Autodesk Inventor part; units mm, degrees
ref_plane "Work Plane1" through (-21.8189, 29, 8.1) normal (0, 1, 0) x (0, 0, 1)
ref_plane "Work Plane2" through (-21.8189, 19, 8.1) normal (0, 0, -1) x (0, 1, 0)
ref_plane "YZ Plane" through (0, 0, 0) normal (1, 0, 0) x (0, 1, 0)
sketch "Sketch1" plane through (0, 0, 0) normal (0, 0, 1) x (1, 0, 0)
  line L0 (5.8439, -14.5) -> (6.8, -14.5)
  line L1 (6.8, -5.5) -> (6.8, -14.5)
  line L2 (6.8, -5.5) -> (5.8439, -5.5)
  arc A0 (5.8439, -3.1) -> (5.8439, -5.5) centre (4, -4.3) ccw
  line L3 (5.8439, -3.1) -> (6.8, -3.1)
  line L4 (6.8, 0) -> (6.8, -3.1)
  line L5 (0, 0) -> (6.8, 0)
  line L6 (0, -20) -> (0, 0)
  line L7 (0, -20) -> (6.8, -20)
  line L8 (6.8, -16.9) -> (6.8, -20)
  line L9 (6.8, -16.9) -> (5.8439, -16.9)
  arc A1 (5.8439, -14.5) -> (5.8439, -16.9) centre (4, -15.7) ccw
  line L10 (-47.1, -14.5) -> (-46.1439, -14.5)
  arc A2 (-46.1439, -16.9) -> (-46.1439, -14.5) centre (-44.3, -15.7) ccw
  line L11 (-46.1439, -16.9) -> (-47.1, -16.9)
  line L12 (-47.1, -16.9) -> (-47.1, -20)
  line L13 (-40.3, -20) -> (-47.1, -20)
  line L14 (-40.3, 0) -> (-40.3, -20)
  line L15 (-40.3, 0) -> (-47.1, 0)
  line L16 (-47.1, 0) -> (-47.1, -3.1)
  line L17 (-47.1, -3.1) -> (-46.1439, -3.1)
  arc A3 (-46.1439, -5.5) -> (-46.1439, -3.1) centre (-44.3, -4.3) ccw
  line L18 (-46.1439, -5.5) -> (-47.1, -5.5)
  line L19 (-47.1, -5.5) -> (-47.1, -14.5)
extrude "Extrusion1" add sketch "Sketch1" along normal blind 4
sketch "Sketch2" plane through (0, 0, 0) normal (0, 1, 0) x (1, 0, 0)
  line L0 (0, 0) -> (6.8, 0)
  line L1 (0, 0) -> (0, -4)
  line L2 (6.8, -4) -> (0, -4)
  line L3 (6.8, 0) -> (6.8, -4)
  line L4 (-47.1, 0) -> (-47.1, -4)
  line L5 (-40.3, -4) -> (-47.1, -4)
  line L6 (6.8, 0) -> (-47.1, 0)
  line L7 (-47.1, 0) -> (-47.1, -4)
  line L8 (-47.1, -4) -> (6.8, -4)
  line L9 (6.8, -4) -> (6.8, 0)
extrude "Extrusion2" add sketch "Sketch2" along normal blind 4 contours L1 L8 L5 L4 L6
sketch "Sketch3" plane through (0, 0, 4) normal (1, 0, 0) x (0, 0, -1)
  line L0 (4, 0) -> (0, 0)
  line L1 (4, 4) -> (4, 0)
  line L2 (0, 4) -> (4, 4)
  line L3 (0, 0) -> (0, 4)
extrude "Extrusion3" add sketch "Sketch3" along normal up to surface (6.8 mm away)
sketch "Sketch4" plane through (0, 4, 0) normal (0, 1, 0) x (1, 0, 0)
  line L0 (6.8, 0) -> (-47.1, 0)
  line L1 (-47.1, -4) -> (6.8, -4)
  line L2 (-9.3767, -8.1) -> (-9.3767, -13.1) construction
  line L3 (-21.8189, -8.1) -> (-9.3767, -8.1) construction
  arc A0 (-17.3767, -8.1) -> (-40.8, 16.4941) centre (-48.3, -14.1) ccw construction
  line L4 (-9.3767, -4) -> (-16.3767, -4) construction
  line L5 (-16.3767, -4) -> (-16.3767, -8.1) construction
  line L6 (-16.3767, -8.1) -> (-9.3767, -8.1) construction
  line L7 (-9.3767, -8.1) -> (-9.3767, -4) construction
  line L8 (-9.3767, -4) -> (-16.3767, -4)
  line L9 (-16.3767, -4) -> (-16.3767, 0)
  line L10 (-16.3767, 0) -> (-9.3767, 0)
  line L11 (-9.3767, 0) -> (-9.3767, -4)
  point P0 (0, 0)
  dimension "d6" = 7
ref_plane "Work Plane1" through (-21.8189, 29, 8.1) normal (0, 1, 0) x (0, 0, 1)
extrude "Extrusion4" add sketch "Sketch4" along normal up to surface (25 mm away)
sketch "Sketch5" plane through (0, 0, 4) normal (0, 0, 1) x (1, 0, 0)
  circle A0 centre (-13.3767, 24) radius 2 construction
  line L0 (-21.8189, 24) -> (-17.3767, 24) construction
  line L1 (-21.8189, 24) -> (-21.8189, 29) construction
  line L2 (-21.8189, 29) -> (-9.3767, 29) construction
  line L3 (-9.3767, 19) -> (-9.3767, 29) construction
  line L4 (-17.3767, 19) -> (-9.3767, 19) construction
  line L5 (-17.3767, 24) -> (-17.3767, 19) construction
  line L6 (-9.3767, 19) -> (-16.3767, 19) construction
  line L7 (-16.3767, 19) -> (-16.3767, 29) construction
  line L8 (-16.3767, 29) -> (-9.3767, 29) construction
  line L9 (-9.3767, 29) -> (-9.3767, 19) construction
  line L10 (-9.3767, 19) -> (-16.3767, 19)
  line L11 (-16.3767, 19) -> (-16.3767, 29)
  line L12 (-16.3767, 29) -> (-9.3767, 29)
  line L13 (-9.3767, 29) -> (-9.3767, 19)
  circle A1 centre (-13.3767, 24) radius 2
ref_plane "Work Plane2" through (-21.8189, 19, 8.1) normal (0, 0, -1) x (0, 1, 0)
extrude "Extrusion5" add sketch "Sketch5" along normal up to surface (4.1 mm away)
fillet "Fillet2" radius 2 2 edges at (-9.3767, 4, 2) (-16.3767, 4, 2)
sketch "Sketch6" plane through (-16.3767, 19, 8.1) normal (-1, 0, 0) x (0, 0, 1)
  line L0 (0, 5) -> (-24.5941, 5) construction
  line L1 (0, 0) -> (-24.5941, 0) construction
  line L2 (-8.1, 10) -> (0.5132, 10) construction
  line L3 (0.5132, 10) -> (0.5132, 5) construction
  line L4 (0.5132, 5) -> (-8.1, 5) construction
  line L5 (-8.1, 5) -> (-8.1, 10) construction
  line L6 (-8.1, 10) -> (0, 10)
  line L7 (0, 10) -> (0, 5)
  line L8 (0, 5) -> (-8.1, 5)
  line L9 (-8.1, 5) -> (-8.1, 10)
  point P0 (-8.1, -19)
extrude "Extrusion6" add sketch "Sketch6" along normal blind 5
sketch "Sketch7" plane through (-16.3767, 24, 0) normal (0, -1, 0) x (1, 0, 0)
  line L0 (0, 8.1) -> (0, 0)
  line L1 (0, 8.1) -> (-5, 8.1)
  line L2 (-5, 0) -> (-5, 8.1)
  line L3 (0, 0) -> (-5, 0)
  point P0 (16.3767, 0)
extrude "Extrusion7" cut sketch "Sketch7" against normal blind 0.4
sketch "Sketch8" plane through (0, 0, 0) normal (0, 0, -1) x (-1, 0, 0)
  circle A0 centre (13.3767, 24) radius 2 construction
  circle A1 centre (13.3767, 24) radius 2
extrude "Extrusion8" cut sketch "Sketch8" against normal blind 4
fillet "Fillet3" radius 1 1 edges at (-16.3767, 24.4, 4.05)
sketch "Sketch9" plane through (-9.3767, 19, 8.1) normal (1, 0, 0) x (0, 0, -1)
  line L0 (0, 0) -> (0, 10)
  line L1 (8.1, 7) -> (0, 7) construction
  line L2 (8.1, 3) -> (0, 3) construction
  line L3 (24.5941, 5) -> (0, 5) construction
  line L4 (-5, 5) -> (0, 5) construction
  line L5 (4, 8.75) -> (7.5, 8.75)
  line L6 (7.5, 8.75) -> (7.5, 1.25)
  line L7 (7.5, 1.25) -> (4, 1.25)
  line L8 (4, 1.25) -> (4, 8.75)
  point P0 (8.1, -19)
  point P1 (4, 5)
  dimension "d20" = 3.5
  dimension "d21" = 7.5
  dimension "d22" = 4
extrude "Extrusion9" cut sketch "Sketch9" against normal blind 7.5
sketch "Sketch10" plane through (-16.3767, 19, 4) normal (0, -1, 0) x (1, 0, 0)
  line L0 (0, 4.1) -> (7, 4.1)
  line L1 (0, 0) -> (0, 4.1)
  line L2 (7, 0) -> (0, 0)
  line L3 (7, 0) -> (7, 4.1)
  point P0 (16.3767, -4)
extrude "Extrusion10" add sketch "Sketch10" along normal blind 3
fillet "Fillet4" radius 3 1 edges at (-12.8767, 16, 4)
sketch "Sketch11" plane through (0, 0, 0) normal (0, -1, 0) x (1, 0, 0)
  line L0 (-40.3, 0) -> (-40.3, 4)
  line L1 (0, 0) -> (-40.3, 0)
  line L2 (0, 0) -> (0, 4)
  line L3 (-40.3, 4) -> (0, 4)
extrude "Extrusion11" cut sketch "Sketch11" against normal blind 0.3
sketch "Sketch12" plane through (0, -20, 0) normal (-1, 0, 0) x (0, 0, 1)
  line L0 (0, 0) -> (0, 20.3)
  line L1 (0, 0) -> (4, 0)
  line L2 (4, 20.3) -> (4, 0)
  line L3 (4, 20.3) -> (0, 20.3)
  point P0 (0, 20)
extrude "Extrusion12" cut sketch "Sketch12" against normal blind 0.3
sketch "Sketch13" plane through (-40.3, -20, 4) normal (1, 0, 0) x (0, 0, -1)
  line L0 (4, 0) -> (4, 20.3)
  line L1 (4, 20.3) -> (0, 20.3)
  line L2 (0, 0) -> (0, 20.3)
  line L3 (4, 0) -> (0, 0)
  point P0 (4, 20)
extrude "Extrusion13" cut sketch "Sketch13" against normal blind 0.3
fillet "Fillet5" radius 1 2 edges at (6.8, 4, 2) (-47.1, 4, 2)
properties part number "MG996RBracket"
Design review of the part built by this model. Coordinates are the model's own, in mm. A direction names the side the tool comes from. Round coordinates to 2 decimals unless told otherwise and drop trailing zeros. Order: outer loops, then holes, each group sorted by start corner. A loop starts at its lowest first (then second) coordinate and runs counter-clockwise, first axis right, second up. Notation, with made-up numbers: M 40,48 L 73,48 A18 ccw 73,52 Z; hole C 30.5,67.25 d11. An arc over 180 degrees is marked long. Put each result on its own line as item: value.
Q1. Insertion check: pin 1 Ø5.5 at (x, y) = (-44.3, -15.7) entering from -Z; pin 2 Ø3.5 at (x, y) = (-13.38, 24) entering from -Z; pin 3 Ø2.5 at (y, z) = (27.5, 4) entering from -X; pin 4 Ø4 at (x, y) = (-4.5, 4) entering from +Z. Each pin has a flat end and moves straight along its axis. Give the tip position at first contact, or say it passes through.
Reported:
pin 1: z = 0
pin 2: through
pin 3: x = -21.38
pin 4: z = 4
Q2. Consider section D-D (x = -13). State the section outline as (y, z) points, and give its area (3 significant figures).
Reported:
outline: M 0.3,0 L 22.04,0 L 22.04,0.6 L 20.25,0.6 L 20.25,4.1 L 22.04,4.1 L 22.04,8.1 L 16,8.1 L 16,7 A3 cw 13,4 L 0.3,4 Z; M 25.96,0 L 29,0 L 29,8.1 L 25.96,8.1 L 25.96,4.1 L 27.75,4.1 L 27.75,0.6 L 25.96,0.6 Z
area: 126 mm²
Q3. Draft analysis for pull direction Y (two halves, no side actions). For faces 1 (the face through (-16.377, 15, 3)), 2 (the face through (6.8, -10, 2)), 3 (the face through (-15, 29, 4)), state which applies: released by +Y, released by -Y, zero draft, split by the parting line, or undercut.
Reported:
face 1: undercut
face 2: zero draft
face 3: released by +Y
Q4. Consider section B-B (x = -19.5). State the section outline as (y, z) points, and give its area (3 significant figures).
Reported:
outline: M 0.3,0 L 4,0 L 4,4 L 0.3,4 Z; M 24.4,0 L 29,0 L 29,8.1 L 24.4,8.1 Z
area: 52.1 mm²
Q5. Consider section A-A (y = -4.3). State the section outline as (x, z) points.
Reported:
outline: M -42.1,0 L -40.6,0 L -40.6,4 L -42.1,4 Z; M 0.3,0 L 1.8,0 L 1.8,4 L 0.3,4 Z
Q6. Machinability: for faces 4 (the face through (-19, 24.4, 4)), 5 (the face through (-40.6, -10, 2)), 6 (the face through (-1, 4, 2)), which of the approach directions +Z, -Z, +X, -X, +Y, -Y give a long, thin tool a straight path to every point of the face, cutting with its end or side? Answer none if there is none.
Reported:
face 4: +Z, -Z, -X
face 5: +Z, -Z, -Y
face 6: +Z, -Z, +X, +Y
Q7. To check wall thickness, follow line 1 (Y direction, x = -44.3, z = 2.4); line 2 (X direction, y = -4.3, z = 2.8); line 3 (X direction, y = -10, z = 2). State the ranges of each line that lie inside material, in increasing order.
Reported:
line 1: -20 to -17.9, -13.5 to -6.5, -2.1 to 4
line 2: -42.1 to -40.6, 0.3 to 1.8
line 3: -47.1 to -40.6, 0.3 to 6.8
Q8. Consider section C-C (x = -44.3). State the section outline as (y, z) points.
Reported:
outline: M -20,0 L -17.9,0 L -17.9,4 L -20,4 Z; M -13.5,0 L -6.5,0 L -6.5,4 L -13.5,4 Z; M -2.1,0 L 4,0 L 4,4 L -2.1,4 Z
